Input: dimensioned drawing with shaded views. Units: mm. Origin: part minimum x, y, z. A direction names the side the tool comes from. Round coordinates to 2 decimals unless told otherwise and drop trailing zeros. Loops run counter-clockwise (first coordinate to the right, second up) from the corner with the lowest first, then second, coordinate; pieces in that order, holes last. Notation, with made-up numbers: (-9.5, 83.25) - (29.5, 83.25) arc R20 cw to (29.5, 117.25) - close; hole circle Ø4 at (49.5, -9). An arc over 180 degrees is marked (long way). Write each question's results on one line, items separated by ' | '.
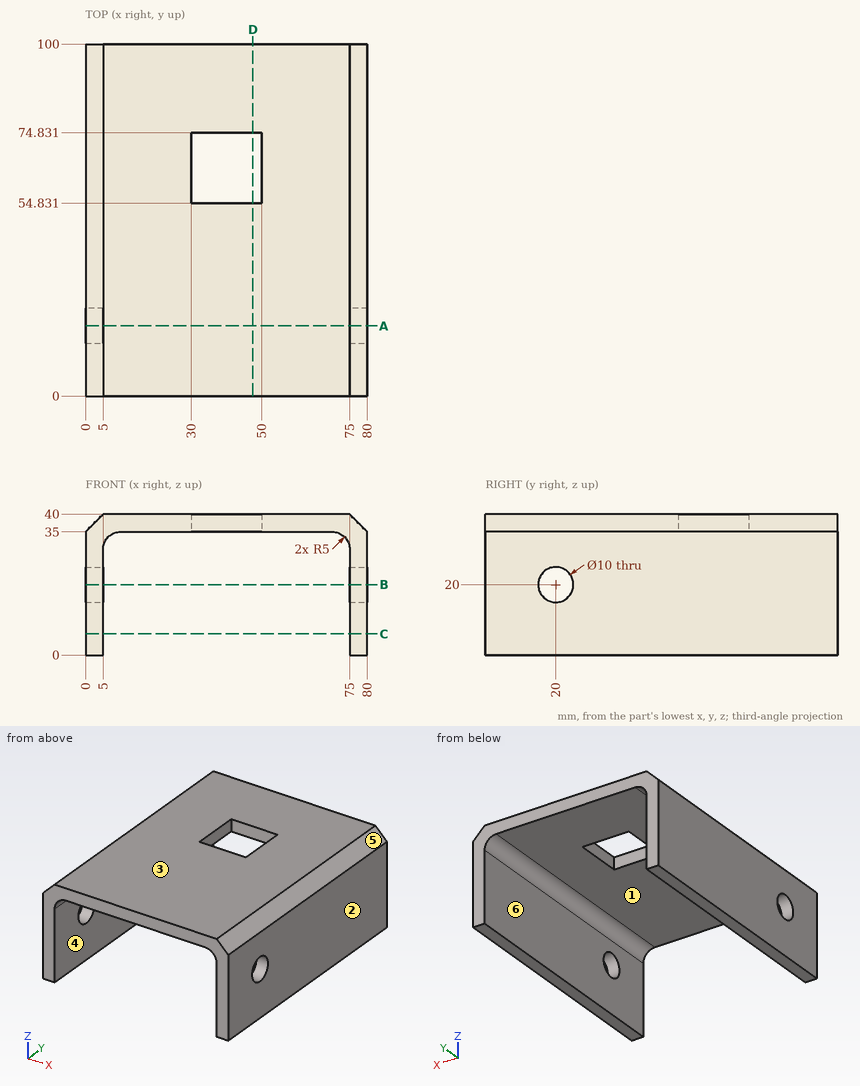
1. Mould query, pull axis X, two halves, no side actions, for the marked faces 1, 2, 3 and 4. Classes: pulls with the +X half, pulls with the -X half, needs draft (parallel to the pull), parting line crosses it, or undercut.
Answer:
face 1: undercut | face 2: pulls with the +X half | face 3: needs draft | face 4: undercut
2. Section query A-A, the plane y = 20. Output: boundary loops of the cut face in (x, z).
Answer:
outline: (0, 0) - (5, 0) - (5, 15) - (0, 15) - close; (0, 25) - (5, 25) - (5, 30) arc R5 cw to (10, 35) - (70, 35) arc R5 cw to (75, 30) - (75, 25) - (80, 25) - (80, 35) - (75, 40) - (5, 40) - (0, 35) - close; (75, 0) - (80, 0) - (80, 15) - (75, 15) - close
3. Set-up query: the marked faces 5 and 6. Return all of +Z, -Z, +X, -X, +Y, -Y with unobstructed straight access to the full face (end or side cutting, diameter ignored); none if empty.
Answer:
face 5: +Z, +X, +Y, -Y | face 6: -Z, +Y, -Y
4. Section query C-C, the plane z = 6. Output: boundary loops of the cut face in (x, y), plus the area to 3 significant figures.
Answer:
outline: (0, 0) - (5, 0) - (5, 100) - (0, 100) - close; (75, 0) - (80, 0) - (80, 100) - (75, 100) - close | area: 1,000 mm^2
5. Contact query for flat-ended pins moving along their axis: pin 1 (1.5 mm diameter, centred on x = 20, y = 48, fed in from -Z); pin 2 (1.5 mm diameter, centred on y = 69, z = 37, fed in from +X); pin 3 (2.5 mm diameter, centred on y = 63.5, z = 38.5, fed in from -X). Output: stop coordinate, or through.
Answer:
pin 1: z = 35 | pin 2: x = 78.75 | pin 3: x = 2.25
6. Section query B-B, the plane z = 20. Output: boundary loops of the cut face in (x, y).
Answer:
outline: (0, 0) - (5, 0) - (5, 15) - (0, 15) - close; (0, 25) - (5, 25) - (5, 100) - (0, 100) - close; (75, 0) - (80, 0) - (80, 15) - (75, 15) - close; (75, 25) - (80, 25) - (80, 100) - (75, 100) - close
7. Section query D-D, the plane x = 47.5. Output: boundary loops of the cut face in (y, z), plus the area to 3 significant figures.
Answer:
outline: (0, 35) - (54.83, 35) - (54.83, 40) - (0, 40) - close; (74.83, 35) - (100, 35) - (100, 40) - (74.83, 40) - close | area: 400 mm^2
8. Line query: line 1 (X direction, y = 39, z = 6); line 2 (Z direction, x = 49.5, y = 46); line 3 (Z direction, x = 2.3, y = 20). Output: solid intervals per line, ascending. Write a range as [from, to].
Answer:
line 1: [0, 5], [75, 80] | line 2: [35, 40] | line 3: [0, 15], [25, 37.3]
